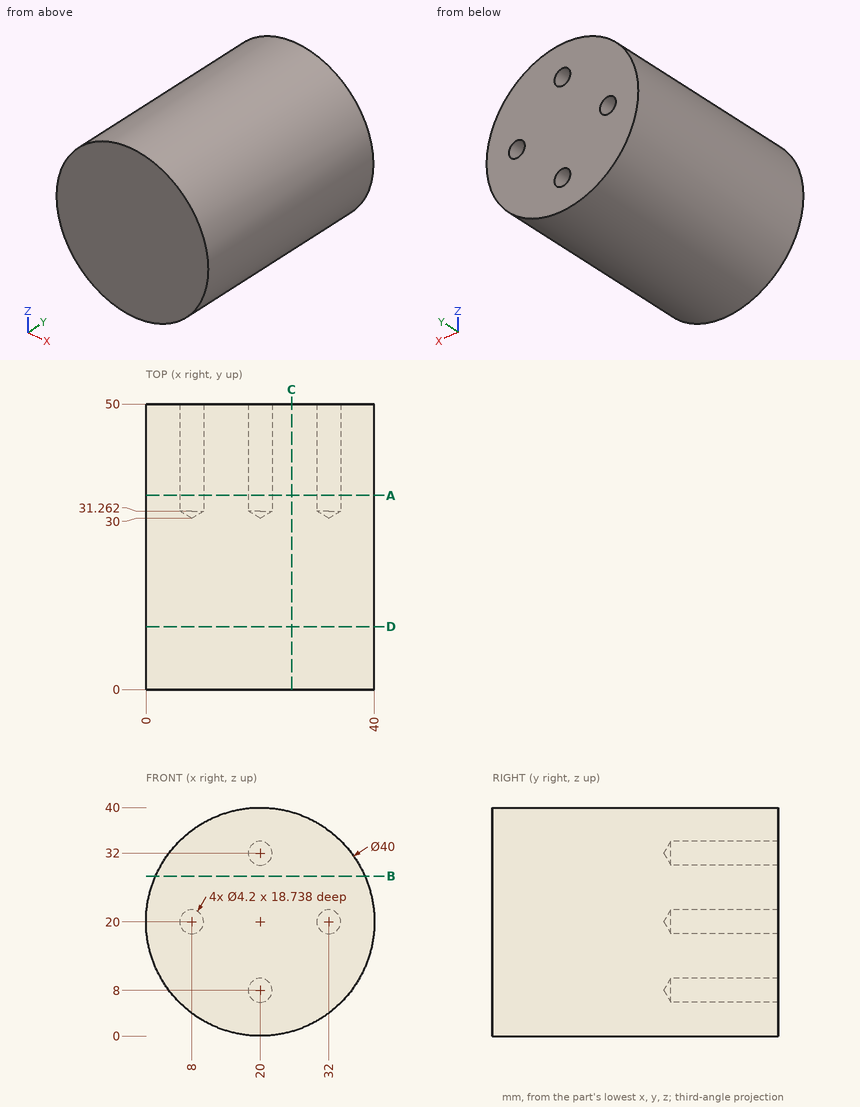
Drawing for the job (mm, zero at the part's lowest x, y, z). Give positions to 0.01 mm unless a question says otherwise; leave off trailing zeros. Write each loop counter-clockwise with the first axis right and the second up, starting at its lowest first coordinate (ties: lowest second). Pieces come first, ordered by that corner, then holes. Notation, with made-up numbers: (-12.75, 46) -> (26.25, 46) arc R28 ccw to (26.25, 75) -> close; hole circle Ø8 at (-37, 26). An arc over 180 degrees is marked (long way). Put each result on its own line as item: value. Start each with the question number.
Item 1: Pin check, flat tips, straight feed: pin 1 Ø12 at (x, y) = (16, 30.5) entering from -Z; pin 2 Ø6 at (x, y) = (7, 21.5) entering from -Z; pin 3 Ø2.5 at (x, z) = (20, 32) entering from +Y. Stop position of each tip, or through.
Item 2: Cut at D-D (y = 11). List the corners of the cut face in (x, z).
Item 3: Cut at B-B (z = 28). List the corners of the cut face in (x, y).
Item 4: Cut at A-A (y = 34). List the corners of the cut face in (x, z).
Item 5: Wall check: L1, parallel to Z at x = 20, y = 41.5; L2, parallel to X at y = 46, z = 20.5. Give the ranges that are in metal, low to high. Write a range as [from, to].
Item 6: Cut at C-C (x = 25.5). List the corners of the cut face in (y, z).
Answer list:
1. pin 1: stops at z = 0
1. pin 2: stops at z = 2.68
1. pin 3: stops at y = 30.75
2. outline: circle Ø40 at (20, 20)
3. outline: (1.67, 0) -> (38.33, 0) -> (38.33, 50) -> (1.67, 50) -> close
4. outline: circle Ø40 at (20, 20); hole circle Ø4.2 at (8, 20); hole circle Ø4.2 at (20, 8); hole circle Ø4.2 at (20, 32); hole circle Ø4.2 at (32, 20)
5. L1: z = [0, 5.9], [10.1, 29.9], [34.1, 40]
5. L2: x = [0.01, 5.96], [10.04, 29.96], [34.04, 39.99]
6. outline: (0, 0.77) -> (50, 0.77) -> (50, 39.23) -> (0, 39.23) -> close
